from build123d import *

# Parameters (mm, degrees)
SKETCH1_W           = 145
SKETCH1_H           = 40
SKETCH1_W_2         = 141
SKETCH1_H_2         = 36
BOSS_EXTRUDE1_DEPTH = 30
SKETCH2_W           = 145
SKETCH2_H           = 40
BOSS_EXTRUDE2_DEPTH = 2
SKETCH3_W           = 153
SKETCH3_H           = 48
SKETCH3_W_2         = 145
SKETCH3_H_2         = 40
BOSS_EXTRUDE3_DEPTH = 4
CHAMFER1_SIZE       = 4
SKETCH4_W           = 20
SKETCH4_H           = 16
SKETCH4_R           = 1.3
BOSS_EXTRUDE4_DEPTH = 10


with BuildPart() as part:
    # Sketch1 → Boss-Extrude1 (new body)
    with BuildSketch(Plane(origin=(0, 0, 0), x_dir=(1, 0, 0), z_dir=(0, 1, 0))):
        Rectangle(SKETCH1_W, SKETCH1_H)
        Rectangle(SKETCH1_W_2, SKETCH1_H_2, mode=Mode.SUBTRACT)
    extrude(amount=BOSS_EXTRUDE1_DEPTH)

    # Sketch2 → Boss-Extrude2 (add)
    with BuildSketch(Plane.XZ):
        Rectangle(SKETCH2_W, SKETCH2_H)
    extrude(amount=BOSS_EXTRUDE2_DEPTH)

    # Sketch3 → Boss-Extrude3 (add)
    with BuildSketch(Plane(origin=(0, 30, 0), x_dir=(1, 0, 0), z_dir=(0, 1, 0))):
        Rectangle(SKETCH3_W, SKETCH3_H)
        Rectangle(SKETCH3_W_2, SKETCH3_H_2, mode=Mode.SUBTRACT)
    extrude(amount=-BOSS_EXTRUDE3_DEPTH)

    # Chamfer1
    chamfer1_edges = [part.edges().sort_by_distance(p)[0] for p in [
        (-72.5, 26, 0),
        (0, 26, 20),
        (72.5, 26, 0),
        (0, 26, -20),
    ]]
    chamfer(chamfer1_edges, length=CHAMFER1_SIZE - 0.0001)  # a hair under: the kernel refuses the full size

    # Sketch4 → Boss-Extrude4 (add)
    # profile 1 of 4: a face of its own
    with BuildSketch(Plane.XZ.offset(2)):
        with Locations((62.5, 28)):
            Rectangle(SKETCH4_W, SKETCH4_H)
        with Locations(Location((62.5, 28, 0), (0, 0, 90))):
            Circle(SKETCH4_R, mode=Mode.SUBTRACT)
    # profile 2 of 4: a face of its own
    with BuildSketch(Plane.XZ.offset(2)):
        with Locations((-62.5, 28)):
            Rectangle(SKETCH4_W, SKETCH4_H)
        with Locations(Location((-62.5, 28, 0), (0, 0, 270))):
            Circle(SKETCH4_R, mode=Mode.SUBTRACT)
    # profile 3 of 4: a face of its own
    with BuildSketch(Plane.XZ.offset(2)):
        with Locations((-62.5, -28)):
            Rectangle(SKETCH4_W, SKETCH4_H)
        with Locations(Location((-62.5, -28, 0), (0, 0, 90))):
            Circle(SKETCH4_R, mode=Mode.SUBTRACT)
    # profile 4 of 4: a face of its own
    with BuildSketch(Plane.XZ.offset(2)):
        with Locations((62.5, -28)):
            Rectangle(SKETCH4_W, SKETCH4_H)
        with Locations(Location((62.5, -28, 0), (0, 0, 270))):
            Circle(SKETCH4_R, mode=Mode.SUBTRACT)
    extrude(amount=-BOSS_EXTRUDE4_DEPTH)


solid = part.part
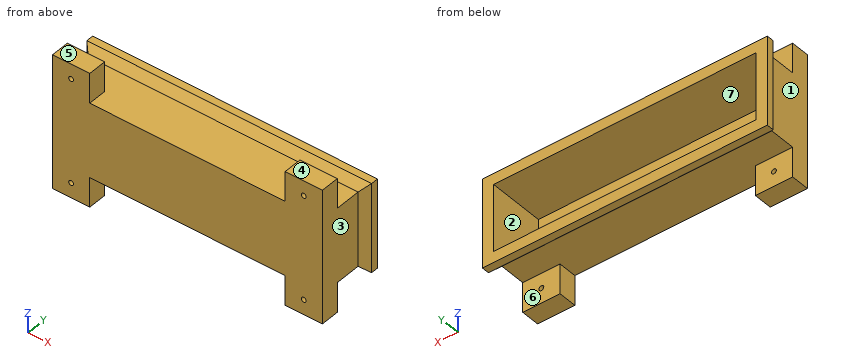
For this review, take the finished solid that the model builds, in its own axes (mm). Face numbers are marked on the shaded views. A direction names the side the tool comes from. Coordinates: 2 decimals unless noted, no trailing zeros. Loops run counter-clockwise (first coordinate to the right, second up) from the corner with the lowest first, then second, coordinate; pieces in that order, holes last. Notation, with made-up numbers: (77.5, -38) - (111.5, -38) arc R21 cw to (111.5, 1) - close; hole circle Ø9 at (28, 8). An arc over 180 degrees is marked (long way). Use a Markdown table: item, result. Add a question column.
Item 1: Mouldability with a two-part tool opening along X and no side actions: class the marked faces 1, 2, 3 and 4 as pulls with the +X half, pulls with the -X half, needs draft (parallel to the pull), parting line crosses it, or undercut.
Item 2: We need section C-C (y = 20). Give the boundary of the cut face in (x, z).
Item 3: For line 1 (X direction, y = 2, z = 28); line 2 (Z direction, x = 12, y = 22); line 3 (X direction, y = 9, z = -14.5), list the stretches that pass through material, from the lowest coordinate up.
Item 4: We need section A-A (y = 6). Give the boundary of the cut face in (x, z), and give its area (3 significant figures).
Item 5: Tool access review of the marked faces 5, 6 and 7: name each direction out of +Z, -Z, +X, -X, +Y, -Y from which nothing blocks a thin tool from reaching the whole face with its end or side.
Item 6: Insertion check: pin 1 Ø7 at (y, z) = (5, -12) entering from -X; pin 2 Ø5 at (x, z) = (-17, 26) entering from -Y; pin 3 Ø5 at (x, y) = (-29, 20) entering from +Z; pin 4 Ø17.5 at (x, z) = (62.5, 26) entering from +Y. Each pin has a flat end and moves straight along its axis. Give the tip position at first contact, or say it passes through.
Results list:
| question | item | result |
|---|---|---|
| 1 | face 1 | pulls with the -X half |
| 1 | face 2 | undercut |
| 1 | face 3 | pulls with the +X half |
| 1 | face 4 | needs draft |
| 2 | outline | (-72.5, -20) - (72.5, -20) - (72.5, 20) - (-72.5, 20) - close; hole (-70.5, -18) - (70.5, -18) - (70.5, 18) - (-70.5, 18) - close |
| 3 | line 1 | x = -72.5 to -63.8, -61.2 to -52.5, 52.5 to 61.2, 63.8 to 72.5 |
| 3 | line 2 | z = -20 to -18, 18 to 20 |
| 3 | line 3 | x = -72.5 to -70.5, 70.5 to 72.5 |
| 4 | outline | (-72.5, -36) - (-52.5, -36) - (-52.5, -20) - (52.5, -20) - (52.5, -36) - (72.5, -36) - (72.5, 36) - (52.5, 36) - (52.5, 20) - (-52.5, 20) - (-52.5, 36) - (-72.5, 36) - close; hole (-70.5, -18) - (70.5, -18) - (70.5, 18) - (-70.5, 18) - close; hole circle Ø2.6 at (-62.5, -28); hole circle Ø2.6 at (-62.5, 28); hole circle Ø2.6 at (62.5, -28); hole circle Ø2.6 at (62.5, 28) |
| 4 | area | 1,980 mm^2 |
| 5 | face 5 | +Z, +X, -X, +Y, -Y |
| 5 | face 6 | -Z, +X, -X |
| 5 | face 7 | +Y |
| 6 | pin 1 | stops at x = -72.5 |
| 6 | pin 2 | stops at y = 25.5 |
| 6 | pin 3 | stops at z = 20.5 |
| 6 | pin 4 | stops at y = 30 |
